Geometry: final body of the model. Coordinates: model frame, mm. A direction names the side the tool comes from. Coordinates: 2 decimals unless noted, no trailing zeros. Write each loop counter-clockwise with the first axis right and the second up, starting at its lowest first coordinate (ties: lowest second). Pieces come first, ordered by that corner, then holes.
from build123d import *

# Parameters (mm, degrees)
SKETCH1_W           = 10
SKETCH1_H           = 4
BOSS_EXTRUDE1_DEPTH = 2
SKETCH2_R           = 1.5
CUT_EXTRUDE1_DEPTH  = 1
SKETCH3_R           = 1
BOSS_EXTRUDE2_DEPTH = 50
BOSS_EXTRUDE3_DEPTH = 4
FILLET1_R           = 0.5
SKETCH6_R           = 1
BOSS_EXTRUDE6_DEPTH = 3
FILLET2_R           = 0.5
SKETCH18_R          = 0.996476916
BOSS_EXTRUDE7_DEPTH = 3


with BuildPart() as part:
    # Sketch1 → Boss-Extrude1 (new body)
    with BuildSketch(Plane.XY):
        with Locations((-90.227807008, -9.049640054)):
            Rectangle(SKETCH1_W, SKETCH1_H)
    extrude(amount=BOSS_EXTRUDE1_DEPTH)

    # Sketch2 → Cut-Extrude1 (cut)
    with BuildSketch(Plane.XY.offset(2)):
        with Locations((-93.279774428, -9.049640054)):
            Circle(SKETCH2_R)
        with Locations((-89.227807008, -9.049640054)):
            Circle(SKETCH2_R)
    extrude(amount=-CUT_EXTRUDE1_DEPTH, mode=Mode.SUBTRACT)

    # Sketch3 → Boss-Extrude2 (add)
    with BuildSketch(Plane(origin=(-85.227807008, 0, 0), x_dir=(0, 0, -1), z_dir=(1, 0, 0))):
        with Locations((-1, -9.054602908)):
            Circle(SKETCH3_R)
    extrude(amount=BOSS_EXTRUDE2_DEPTH)

    # Sketch4 → Boss-Extrude3 (add)
    with BuildSketch(Plane(origin=(0, -7.049640054, 0), x_dir=(1, 0, 0), z_dir=(0, 1, 0))):
        Polygon((-35.238104557, 0), (-35.238104557, 2), (-31.238104557, 2), (-31.238104557, 0), (-34.367083254, 0), (-34.367083254, -2.010361564), (-31.238104557, -2.010361564), (-31.238104557, -4.010361564), (-35.238104557, -4.010361564), align=None)
    extrude(amount=-BOSS_EXTRUDE3_DEPTH)

    # Fillet1
    fillet1_edges = [part.edges().sort_by_distance(p)[0] for p in [
        (-35.238104557, -11.049640054, 1.005180782),
        (-35.238104557, -9.049640054, 4.010361564),
        (-33.238104557, -11.049640054, -2),
        (-35.238104557, -9.049640054, -2),
        (-31.238104557, -9.049640054, -2),
        (-33.238104557, -11.049640054, 4.010361564),
        (-35.238104557, -7.049640054, 1.005180782),
        (-33.238104557, -7.049640054, 4.010361564),
        (-33.238104557, -7.049640054, -2),
    ]]
    fillet(fillet1_edges, radius=FILLET1_R)

    # Sketch6 → Boss-Extrude6 (add)
    with BuildSketch(Plane(origin=(0, 0, -2), x_dir=(-1, 0, 0), z_dir=(0, 0, -1))):
        with Locations((33.238104557, -9.038134052)):
            Circle(SKETCH6_R)
    extrude(amount=BOSS_EXTRUDE6_DEPTH)

    # Sketch16 → Revolve10 (revolve)
    with BuildSketch(Plane(origin=(0, 0, -5), x_dir=(-1, 0, 0), z_dir=(0, 0, -1))):
        with BuildLine():
            Line((33.238104557, -7.549640054), (33.238104557, -10.549640054))
            ThreePointArc((33.238104557, -10.549640054), (34.738104557, -9.049640054), (33.238104557, -7.549640054))
        make_face()
    revolve(axis=Axis((-33.238104557, -1009.038134052, -5), (0, 1, 0)))

    # Fillet2
    fillet2_edges = [part.edges().sort_by_distance(p)[0] for p in [
        (-31.238104557, -11.049640054, 2.760361564),
        (-31.238104557, -7.049640054, 2.760361564),
        (-31.238104557, -9.049640054, 4.010361564),
        (-31.238104557, -7.196086663, 3.863914954),
        (-31.238104557, -10.903193444, 3.863914954),
    ]]
    fillet(fillet2_edges, radius=FILLET2_R)

    # Sketch18 → Boss-Extrude7 (add)
    with BuildSketch(Plane.XY.offset(4.010361564)):
        with Locations((-33.23429851, -9.03071029)):
            Circle(SKETCH18_R)
    extrude(amount=BOSS_EXTRUDE7_DEPTH)

    # Sketch20 → Revolve22 (revolve)
    with BuildSketch(Plane.XY.offset(7.010361564)):
        with BuildLine():
            Line((-33.23429851, -7.550711674), (-33.23429851, -10.510708905))
            ThreePointArc((-33.23429851, -10.510708905), (-31.754299895, -9.03071029), (-33.23429851, -7.550711674))
        make_face()
    revolve(axis=Axis((-33.23429851, -1009.03071029, 7.010361564), (0, 1, 0)))


solid = part.part
Item 1: Section B-B, the plane x = -38. Output: boundary loops of the cut face in (y, z).
Derived:
outline: circle Ø2 at (-9.05, 1)
Item 2: Pin query (flat end, axial travel): pin 1 (8 mm diameter, centred on x = -43.5, z = -1, fed in from +Y); pin 2 (0.9 mm diameter, centred on x = -93, y = -9.5, fed in from +Z); pin 3 (1.8 mm diameter, centred on x = -93.28, y = -9.05, fed in from -Z). Return the tip coordinate at first contact, or that it passes through.
Derived:
pin 1: stops at y = -8.05
pin 2: stops at z = 1
pin 3: stops at z = 0
Item 3: Section A-A, the plane z = -0.75. Output: boundary loops of the cut face in (x, y), plus the area to 3 significant figures.
Derived:
outline: (-35.24, -10.55) arc R0.5 ccw to (-34.74, -11.05) - (-31.24, -11.05) - (-31.24, -7.05) - (-34.74, -7.05) arc R0.5 ccw to (-35.24, -7.55) - close
area: 15.9 mm2
Item 4: Pull-direction query (X, two-part tool) for faces 1 (the flat face through (-90, -11.05, 1)), 2 (the flat face through (-31.238, -9, -1)), 3 (the cylindrical face through (-34.23, -8.99, 4.95)), 4 (the flat face through (-35.238, -8, 0)); classes: released by +X, released by -X, zero draft, split by the parting line, or undercut.
Derived:
face 1: zero draft
face 2: released by +X
face 3: split by the parting line
face 4: undercut
Item 5: Material intervals for probe 1 along X at (y, z) = (-9.65, 3); probe 2 along X at (y, z) = (-7.15, 0.5); probe 3 along X at (y, z) = (-9, 0.25), sorted ascending.
Derived:
probe 1: x = -35.24 to -31.24
probe 2: x = -95.23 to -85.23, -35.04 to -34.37
probe 3: x = -95.23 to -34.37
Item 6: Set-up query: faces 5 (the flat face through (-34.367, -9, 1)), 6 (the cylindrical face through (-90.42, -9.96, 1.51)), 7 (the flat face through (-85.228, -7.6, 1)). Return all of +Z, -Z, +X, -X, +Y, -Y with unobstructed straight access to the full face (end or side cutting, diameter ignored); none if empty.
Derived:
face 5: +X, +Y, -Y
face 6: +Z
face 7: +Y
